Check sheet for the modelled part. Datum: model origin and axes. Units: mm. Round coordinates to 2 decimals unless told otherwise and drop trailing zeros. Loops run counter-clockwise (first coordinate to the right, second up) from the corner with the lowest first, then second, coordinate; pieces in that order, holes last. Notation, with made-up numbers: (86.5, 19.25) - (143.5, 19.25) arc R16 cw to (143.5, 30.25) - close; hole circle Ø9 at (85, 86.25). An arc over 180 degrees is marked (long way). Put each result on its own line as item: value. Start each with the question number.
Item 1: Material ranges on line 1 along X through (y, z) = (0.35, 12); line 2 along Z through (x, y) = (5, 0.4); line 3 along Z through (x, y) = (-5.5, 0.9), recorded low to high.
Item 2: Section check A-A, the plane z = -4. Record the cut outline in (x, y), and give its area (3 significant figures).
Item 3: Section check D-D, the plane z = 7. Record the cut outline in (x, y), and give its area (3 significant figures).
Item 4: Section check C-C, the plane z = 11.5. Record the cut outline in (x, y), and give its area (3 significant figures).
Item 5: Section check B-B, the plane y = 1.1. Record the cut outline in (x, z), and give its area (3 significant figures).
from build123d import *

# Parameters (mm, degrees)
SKETCH_1_R      = 0.95
EXTRUDE_1_DEPTH = 1.3


with BuildPart() as part:
    # 草图1 → 凸台-拉伸1 (new body)
    with BuildSketch(Plane(origin=(0, 0, 0), x_dir=(1, 0, 0), z_dir=(0, 1, 0))):
        with BuildLine():
            ThreePointArc((6.366785174, -10.348273625), (4.336586912, -10.567387921), (3.744794787, -12.521741558))
            Line((3.744794787, -12.521741558), (4.570066616, -15.281262746))
            ThreePointArc((4.570066616, -15.281262746), (0, 15.95), (-4.570066616, -15.281262746))
            Line((-4.570066616, -15.281262746), (-3.744794792, -12.521741574))
            ThreePointArc((-3.744794792, -12.521741574), (-4.336586905, -10.567387926), (-6.366785174, -10.348273625))
            ThreePointArc((-6.366785174, -10.348273625), (-8.87577758, -10.671754493), (-11.00617365, -9.30753481))
            ThreePointArc((-11.00617365, -9.30753481), (0, 12.95), (11.00617365, -9.30753481))
            ThreePointArc((11.00617365, -9.30753481), (8.87577758, -10.671754493), (6.366785174, -10.348273625))
        make_face()
        with Locations(Location((5.517229655, -11.991671149, 0), (0, 0, 270))):
            Circle(SKETCH_1_R, mode=Mode.SUBTRACT)
        with Locations(Location((-5.517229655, -11.991671149, 0), (0, 0, 270))):
            Circle(SKETCH_1_R, mode=Mode.SUBTRACT)
    extrude(amount=EXTRUDE_1_DEPTH)


solid = part.part
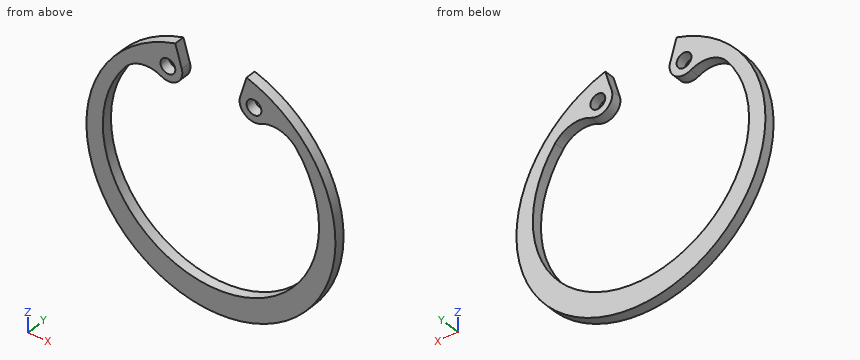
Check result:
1. line 1: -10.51 to -6.47, -4.57 to -3.67, 3.67 to 4.57, 6.47 to 10.51
1. line 2: -15.15 to -12.02, 10.22 to 11.19, 12.79 to 15.15
1. line 3: -14.97 to -11.81, 10.14 to 11.04, 12.94 to 14.97
2. outline: (-15.44, 0) - (-12.95, 0) - (-12.95, 1.3) - (-15.44, 1.3) - close; (12.95, 0) - (15.44, 0) - (15.44, 1.3) - (12.95, 1.3) - close
2. area: 6.46 mm²
3. outline: (-14.33, 0) - (-12.43, 0) - (-12.43, 1.3) - (-14.33, 1.3) - close; (12.43, 0) - (14.33, 0) - (14.33, 1.3) - (12.43, 1.3) - close
3. area: 4.93 mm²
4. outline: (-11.05, 0) - (-6.33, 0) - (-6.33, 1.3) - (-11.05, 1.3) - close; (-4.7, 0) - (-3.73, 0) - (-3.73, 1.3) - (-4.7, 1.3) - close; (3.73, 0) - (4.7, 0) - (4.7, 1.3) - (3.73, 1.3) - close; (6.33, 0) - (11.05, 0) - (11.05, 1.3) - (6.33, 1.3) - close
4. area: 14.8 mm²
5. outline: (-11.01, 9.31) arc R3.7 cw to (-6.37, 10.35) arc R1.85 ccw to (-3.74, 12.52) - (-4.57, 15.28) arc R15.95 ccw (long way) to (4.57, 15.28) - (3.74, 12.52) arc R1.85 ccw to (6.37, 10.35) arc R3.7 cw to (11.01, 9.31) arc R13.85 cw (long way) to start; hole circle Ø1.9 at (-5.52, 11.99); hole circle Ø1.9 at (5.52, 11.99)
5. area: 207 mm²
